Could you check a few things on this drawing? It's one solid part, dimensions in mm from its lowest x, y, z. Give positions to 0.01 mm unless a question says otherwise; leave off trailing zeros. Write each loop counter-clockwise with the first axis right and the second up, starting at its lowest first coordinate (ties: lowest second). Pieces come first, ordered by that corner, then holes. Notation, with made-up numbers: (73, -19.5) -> (110, -19.5) arc R5 ccw to (110, -11.5) -> close; hole circle Ø11 at (35.25, -22). An arc over 180 degrees is marked (long way). Use CSV: the item, a comma, the result in double quotes. Start each with the question number.
(1) For pin 1 Ø1.5 at (y, z) = (3, 6.5) entering from -X, with a flat end and sliding along its axis, tell me the tip position at first contact or that it passes through.
(2) I need wall thicknesses on L1, parallel to X at y = 2.55, z = 14.5; L2, parallel to X at y = 0.2, z = 12.5 (1 decimal); L3, parallel to X at y = 3, z = 6.75 (1 decimal). Which ranges of each line are inside material? Lowest first, please. Write a range as [from, to].
(3) Suppose I cut it at A-A on y = 2.4. List the corners of the cut face in (x, z) for me.
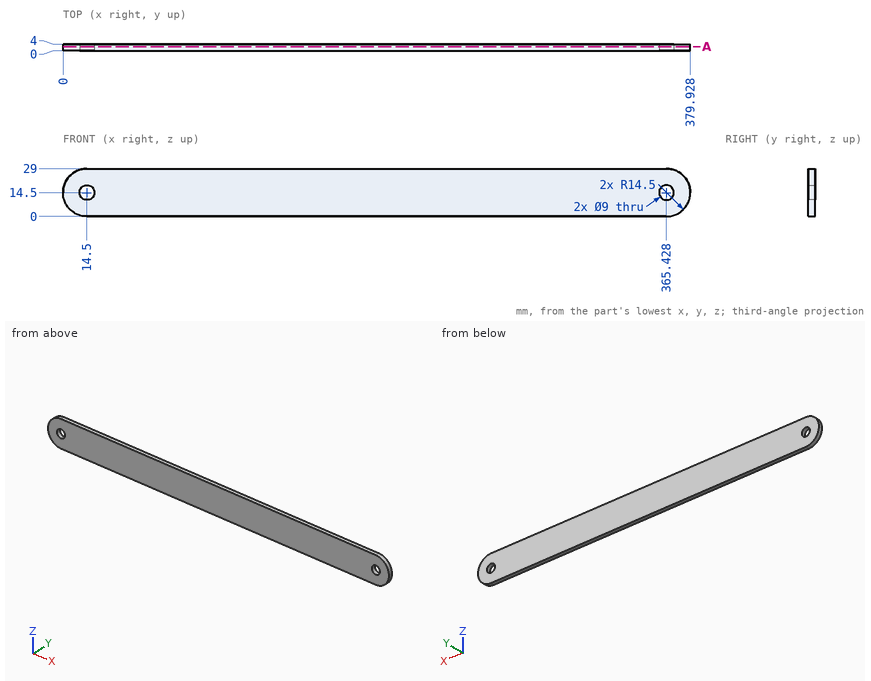
Geometry says:
1,pin 1,"x = 1.94"
2,L1,"[0, 10], [19, 360.93], [369.93, 379.93]"
2,L2,"[0.1, 10.5], [18.5, 361.4], [369.5, 379.8]"
2,L3,"[2.2, 377.7]"
3,outline,"(14.5, 0) -> (365.43, 0) arc R14.5 ccw to (365.43, 29) -> (14.5, 29) arc R14.5 ccw to start; hole circle Ø9 at (14.5, 14.5); hole circle Ø9 at (365.43, 14.5)"
